from build123d import *

# Parameters (mm, degrees)
F0_R     = 9.525
F1_DEPTH = 203.2
F2_W     = 19.05
F2_H     = 25.4
F3_DEPTH = 25.4
F4_R     = 4.7625
F5_DEPTH = 19.051


with BuildPart() as f1:
    # F0 (on Top) → F1 (new body)
    with BuildSketch(Plane.XY):
        Circle(F0_R)
    extrude(amount=F1_DEPTH)

    # F2 (on face) → F3 (join)
    with BuildSketch(Plane.XY.offset(203.2)):
        Rectangle(F2_W, F2_H)
    extrude(amount=F3_DEPTH)

    # F4 (on face) → F5 (cut, through all)
    with BuildSketch(Plane.YZ.offset(9.525)):
        with Locations((0, 222.25)):
            Circle(F4_R)
    extrude(amount=-F5_DEPTH, mode=Mode.SUBTRACT)


solid = f1.part
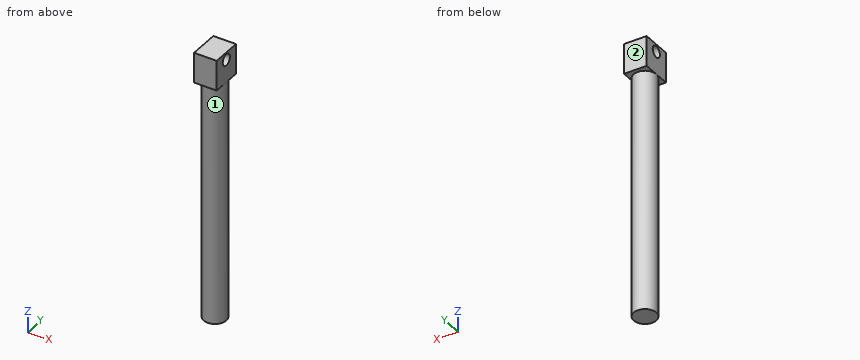
Input: part model. Units: mm. Frame: model coordinates. Face numbers are marked on the shaded views. A direction names the side the tool comes from. Coordinates: 2 decimals unless noted, no trailing zeros. Loops run counter-clockwise (first coordinate to the right, second up) from the corner with the lowest first, then second, coordinate; pieces in that order, holes last.
(1) First-contact query: pin 1 Ø7.5 at (y, z) = (0, 222.25) entering from +X; pin 2 Ø1 at (x, z) = (-2, 95.5) entering from -Y; pin 3 Ø3 at (x, z) = (-1.5, 136) entering from -Y (3 decimals); pin 4 Ø1 at (x, y) = (-2, -5.5) entering from -Z. Flat tips, straight axial feed; report the tip coordinate or a pass-through.
(2) Set-up query: the marked faces 1 and 2. Return all of +Z, -Z, +X, -X, +Y, -Y with unobstructed straight access to the full face (end or side cutting, diameter ignored); none if empty.
(3) Section D-D on y = 6.75. Return the cut outline in (x, z) (3 decimals).
(4) Section C-C on y = -2.5. Return the cut outline in (x, z) (3 decimals), then the cut area to 3 significant figures.
(5) Section A-A on z = 222.25. Return the cut outline in (x, y) (1 decimal).
(6) Material intervals for probe 1 along Z at (x, y) = (-0.5, 0); probe 2 along Z at (x, y) = (3, -11.5); probe 3 along Y at (x, z) = (0.5, 170), sorted ascending.
Data:
1. pin 1: passes through
1. pin 2: stops at y = -9.41
1. pin 3: stops at y = -9.525
1. pin 4: stops at z = 0
2. face 1: -Z
2. face 2: +Z, -Z, +X, -X, +Y
3. outline: (-9.525, 203.2) - (-6.72, 203.2) - (-6.72, 0) - (6.72, 0) - (6.72, 203.2) - (9.525, 203.2) - (9.525, 228.6) - (-9.525, 228.6) - close
4. outline: (-9.525, 203.2) - (-9.191, 203.2) - (-9.191, 0) - (9.191, 0) - (9.191, 203.2) - (9.525, 203.2) - (9.525, 218.196) - (-9.525, 218.196) - close; (-9.525, 226.304) - (9.525, 226.304) - (9.525, 228.6) - (-9.525, 228.6) - close
4. area: 4,060 mm2
5. outline: (-9.5, -12.7) - (9.5, -12.7) - (9.5, -4.8) - (-9.5, -4.8) - close; (-9.5, 4.8) - (9.5, 4.8) - (9.5, 12.7) - (-9.5, 12.7) - close
6. probe 1: z = 0 to 217.49, 227.01 to 228.6
6. probe 2: z = 203.2 to 228.6
6. probe 3: y = -9.51 to 9.51
